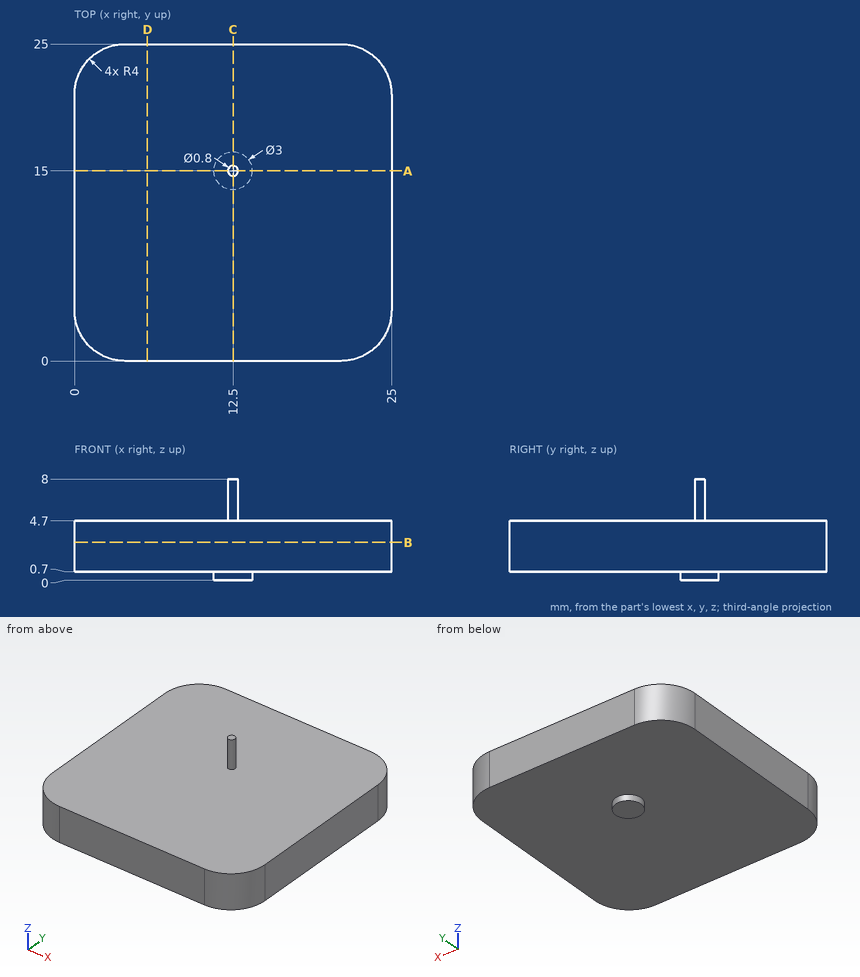
Check sheet for the drawn part. Datum: minimum x, y, z corner. Units: mm. Give positions to 0.01 mm unless a question says otherwise; leave off trailing zeros. Write each loop counter-clockwise with the first axis right and the second up, starting at its lowest first coordinate (ties: lowest second). Pieces come first, ordered by that corner, then holes.
(1) Material ranges on line 1 (Z direction, x = 11, y = 16.5); line 2 (Y direction, x = 23, z = 4.25); line 3 (Y direction, x = 23.75, z = 2), recorded low to high.
(2) Gauge pin test, flat ends, axial feed: pin 1 (7.5 mm diameter, centred on x = 17, y = 15.5, fed in from +Z); pin 2 (1.5 mm diameter, centred on x = 21, y = 15, fed in from -Z). Record the tip position at first contact, or that the pin passes through.
(3) Cross-section at B-B (z = 3). Enter the section's corners in (x, y).
(4) Cross-section at A-A (y = 15). Enter the section's corners in (x, z), plus the area to 3 significant figures.
(5) Cross-section at D-D (x = 5.75). Enter the section's corners in (y, z), plus the area to 3 significant figures.
(6) Cross-section at C-C (x = 12.5). Enter the section's corners in (y, z), plus the area to 3 significant figures.
Worked out:
1. line 1: z = 0.7 to 4.7
1. line 2: y = 0.54 to 24.46
1. line 3: y = 1.1 to 23.9
2. pin 1: stops at z = 4.7
2. pin 2: stops at z = 0.7
3. outline: (0, 4) arc R4 ccw to (4, 0) - (21, 0) arc R4 ccw to (25, 4) - (25, 21) arc R4 ccw to (21, 25) - (4, 25) arc R4 ccw to (0, 21) - close
4. outline: (0, 0.7) - (11, 0.7) - (11, 0) - (14, 0) - (14, 0.7) - (25, 0.7) - (25, 4.7) - (12.9, 4.7) - (12.9, 8) - (12.1, 8) - (12.1, 4.7) - (0, 4.7) - close
4. area: 105 mm2
5. outline: (0, 0.7) - (25, 0.7) - (25, 4.7) - (0, 4.7) - close
5. area: 100 mm2
6. outline: (0, 0.7) - (13.5, 0.7) - (13.5, 0) - (16.5, 0) - (16.5, 0.7) - (25, 0.7) - (25, 4.7) - (15.4, 4.7) - (15.4, 8) - (14.6, 8) - (14.6, 4.7) - (0, 4.7) - close
6. area: 105 mm2
